Work out the finished part from the listing and answer in its coordinate system (mm). A direction names the side the tool comes from. Round coordinates to 2 decimals unless told otherwise and drop trailing zeros. Write each loop counter-clockwise with the first axis right and the second up, starting at its lowest first coordinate (ties: lowest second). Pieces come first, ordered by that corner, then holes.
1. A tool of negligible diameter and unlimited length cuts with its end or side. For faces 4 (the face through (-8.22, -54.25, 17.05)), 5 (the face through (5, -12, 10)), 6 (the face through (3, -33, 5.825)), 7 (the face through (10.07, -23.601, 13.605)), from which of +Z, -Z, +X, -X, +Y, -Y can it reach the whole face along a straight path? Write none if from no direction.
2. Find section B-B (x = -1.75). Write down the section's boundary in (y, z) (3 decimals), and give its area (3 significant figures).
3. Find section C-C (z = 10). Count the separate pieces of the cut face and the enclosed holes in it, and give its area (3 significant figures).
4. Flat-ended cylindrical pins translate along their axes: pin 1 Ø4 at (y, z) = (-57, 3) entering from -X; pin 2 Ø5 at (x, y) = (11.5, -12.5) entering from -Z; pin 3 Ø2.5 at (y, z) = (-57, 10.5) entering from -X; pin 4 Ø3.5 at (x, z) = (8.5, 10.5) entering from -Y. Find the tip coordinate at first contact, or state that the pin passes through.
5. Find section A-A (y = -24). Write down the section's boundary in (x, z) (3 decimals), and give its area (3 significant figures).
6. Determine the mould class of faces 1 (the face through (3, -33, 0)), 2 (the face through (-9, -21, 17)), 3 (the face through (10.07, -55.399, 13.605)) for opening direction Z: pulls with the +Z half, pulls with the -Z half, needs draft (parallel to the pull), parting line crosses it, or undercut.
7. Find section D-D (y = -50). Write down the section's boundary in (x, z) (3 decimals).
8. Straight lines are drawn through the part: probe 1 along Z at (x, y) = (8.2, -3); probe 2 along Z at (x, y) = (4.75, -46) (3 decimals); probe 3 along Y at (x, z) = (-7.5, 16.5). For each, find the intervals that lie inside material, in ascending order.
```python
from build123d import *

# Parameters (mm, degrees)
SKETCH_1_R          = 1.7
EXTRUDE_1_DEPTH     = 20
SKETCH_2_W          = 31.643510299
SKETCH_2_H          = 8.35
CUT_EXTRUDE_1_DEPTH = 75.850374033
SKETCH_4_R          = 1.7
CUT_EXTRUDE_3_DEPTH = 73.237455658
FILLET_1_R          = 0.5
FILLET_2_R          = 2
SKETCH_5_W          = 3.571488154
SKETCH_5_H          = 19.286036032
CUT_EXTRUDE_4_DEPTH = 75.850374033
FILLET_3_R          = 1.5
SKETCH_6_W          = 14.583576629
SKETCH_6_H          = 57.679533687
CUT_EXTRUDE_5_DEPTH = 75.850374033
FILLET_4_R          = 10
SKETCH_7_W          = 8.35
SKETCH_7_H          = 33
CUT_EXTRUDE_6_DEPTH = 71.370448485
FILLET_5_R          = 2


# Some blends are built 0.0001 mm under size
with BuildPart() as part:
    # 草图1 → 凸台-拉伸1 (new body)
    with BuildSketch(Plane.XY):
        with BuildLine():
            Line((0, 0), (10, 0))
            Line((10, 0), (10, -15))
            Line((10, -15), (29.096021943, -15))
            Line((29.096021943, -15), (29.096021943, -66))
            Line((29.096021943, -66), (-11.5, -66))
            Line((-11.5, -66), (-11.5, -54.4))
            ThreePointArc((-11.5, -54.4), (0.333421668, -43.75703287), (-9, -30.865568342))
            Line((-9, -30.865568342), (-9, -9.911704997))
            Line((-9, -9.911704997), (-7.763036189, -9.911704997))
            Line((-7.763036189, -9.911704997), (0, -4.543101007))
            Line((0, -4.543101007), (0, 0))
        make_face()
        with Locations((19.5, -30.6)):
            Circle(SKETCH_1_R, mode=Mode.SUBTRACT)
        with Locations((19.5, -56)):
            Circle(SKETCH_1_R, mode=Mode.SUBTRACT)
    extrude(amount=EXTRUDE_1_DEPTH)

    # 草图2 → 切除-拉伸1 (cut, through all)
    with BuildSketch(Plane(origin=(0, 0, 0), x_dir=(1, 0, 0), z_dir=(0, 1, 0))):
        with Locations((-10.82175515, -10)):
            Rectangle(SKETCH_2_W, SKETCH_2_H)
    extrude(amount=-CUT_EXTRUDE_1_DEPTH, mode=Mode.SUBTRACT)

    # 草图4 → 切除-拉伸3 (cut, through all)
    with BuildSketch(Plane(origin=(10, 0, 0), x_dir=(0, 0, -1), z_dir=(1, 0, 0))):
        with Locations(Location((-10, -3, 0), (0, 0, 90))):
            Circle(SKETCH_4_R)
        with Locations(Location((-10, -10, 0), (0, 0, 90))):
            Circle(SKETCH_4_R)
    extrude(amount=-CUT_EXTRUDE_3_DEPTH, mode=Mode.SUBTRACT)

    # 圆角1
    fillet_1_edges = [part.edges().sort_by_distance(p)[0] for p in [
        (-11.5, -66, 17.0875),
        (-9, -30.865568342, 17.0875),
        (-11.5, -66, 2.9125),
        (-9, -30.865568342, 2.9125),
    ]]
    fillet(fillet_1_edges, radius=FILLET_1_R)

    # 圆角2
    # the kernel refuses this fillet: 2 mm, written as the material it adds along each edge
    with BuildSketch(Plane(origin=(0, -4.543101007, 14.175), x_dir=(0, 1, 0), z_dir=(0, 0, 1)), Plane(origin=(0, -4.543101007, 0), x_dir=(0, 1, 0), z_dir=(0, 0, 1))) as fillet_2_piece_1:
        with BuildLine():
            CenterArc((FILLET_2_R * 0.524275273185, FILLET_2_R), FILLET_2_R, 214.666177241, 55.333822759)
            Line((-FILLET_2_R * 0.298204680815, FILLET_2_R * 0.431205902572), (0, 0))
            Line((0, 0), (FILLET_2_R * 0.524275273185, 0))
        make_face()
    extrude(amount=5.825)
    with BuildSketch(Plane(origin=(10, -15, 0), x_dir=(1, 0, 0), z_dir=(0, 0, 1))) as fillet_2_piece_2:
        with BuildLine():
            CenterArc((FILLET_2_R, FILLET_2_R), FILLET_2_R, 180, 90)
            Line((0, FILLET_2_R), (0, 0))
            Line((0, 0), (FILLET_2_R, 0))
        make_face()
    extrude(amount=20)
    # the kernel refuses this fillet: 2 mm, written as the material it takes off along each edge
    with BuildSketch(Plane(origin=(-9, -9.911704997, -4.621806853), x_dir=(0, -1, 0), z_dir=(0, 0, 1)), Plane(origin=(-9, -9.911704997, 9.553193147), x_dir=(0, -1, 0), z_dir=(0, 0, 1))) as fillet_2_2_piece_1:
        with BuildLine():
            CenterArc((1.848722741, 2), FILLET_2_R, 202.427748684, 67.572251316)
            Line((0, 1.236963811), (0, 0))
            Line((0, 0), (1.848722741, 0))
        make_face()
    extrude(amount=15.068613706, mode=Mode.SUBTRACT)
    with BuildSketch(Plane(origin=(0, 0, -5), x_dir=(1, 0, 0), z_dir=(0, 0, 1)), Plane(origin=(0, 0, 9.175), x_dir=(1, 0, 0), z_dir=(0, 0, 1))) as fillet_2_2_piece_2:
        with BuildLine():
            CenterArc((FILLET_2_R, -FILLET_2_R), FILLET_2_R, 90, 90)
            Line((0, -FILLET_2_R), (0, 0))
            Line((0, 0), (FILLET_2_R, 0))
        make_face()
    extrude(amount=15.825, mode=Mode.SUBTRACT)
    with BuildSketch(Plane(origin=(29.096021943, -15, -5), x_dir=(0, -1, 0), z_dir=(0, 0, 1)), Plane(origin=(29.096021943, -66, -5), x_dir=(-1, 0, 0), z_dir=(0, 0, 1))) as fillet_2_2_piece_3:
        with BuildLine():
            CenterArc((FILLET_2_R, -FILLET_2_R), FILLET_2_R, 90, 90)
            Line((0, -FILLET_2_R), (0, 0))
            Line((0, 0), (FILLET_2_R, 0))
        make_face()
    extrude(amount=30, mode=Mode.SUBTRACT)

    # 草图5 → 切除-拉伸4 (cut, through all)
    with BuildSketch(Plane.XY.offset(20)):
        with Locations((-10.285744077, -57.827803492)):
            Rectangle(SKETCH_5_W, SKETCH_5_H)
    extrude(amount=-CUT_EXTRUDE_4_DEPTH, mode=Mode.SUBTRACT)

    # 圆角3
    fillet_3_edges = [part.edges().sort_by_distance(p)[0] for p in [
        (-8.5, -54.015641537, 2.9125),
        (-8.5, -66, 2.9125),
        (-8.5, -54.015641537, 17.0875),
        (-8.5, -66, 17.0875),
    ]]
    fillet(fillet_3_edges, radius=FILLET_3_R)

    # 草图6 → 切除-拉伸5 (cut, through all)
    with BuildSketch(Plane(origin=(0, 0, 0), x_dir=(-1, 0, 0), z_dir=(0, 0, -1))):
        with Locations((-22.291788315, -40.000125123)):
            Rectangle(SKETCH_6_W, SKETCH_6_H)
    extrude(amount=-CUT_EXTRUDE_5_DEPTH, mode=Mode.SUBTRACT)

    # 圆角4
    fillet_4_edges = [part.edges().sort_by_distance(p)[0] for p in [
        (15, -66, 10),
        (15, -15, 10),
    ]]
    fillet(fillet_4_edges, radius=FILLET_4_R - 0.0001)  # a hair under: the kernel refuses the full size

    # 草图7 → 切除-拉伸6 (cut, through all)
    with BuildSketch(Plane.ZY.offset(-5)):
        with Locations((10, -39.5)):
            Rectangle(SKETCH_7_W, SKETCH_7_H)
    extrude(amount=-CUT_EXTRUDE_6_DEPTH, mode=Mode.SUBTRACT)

    # 圆角5
    fillet_5_edges = [part.edges().sort_by_distance(p)[0] for p in [
        (10, -56, 5.825),
        (10, -23, 5.825),
        (10, -23, 14.175),
        (10, -56, 14.175),
    ]]
    fillet(fillet_5_edges, radius=FILLET_5_R)


solid = part.part
```
Worked answers:
1. face 4: +Z, -Z, -X
1. face 5: -X, +Y, -Y
1. face 6: -X
1. face 7: +X, -X
2. outline: (-66, 0) - (-49.323, 0) - (-49.323, 5.825) - (-66, 5.825) - close; (-66, 14.175) - (-49.323, 14.175) - (-49.323, 20) - (-66, 20) - close; (-35.677, 0) - (-5.753, 0) - (-5.753, 5.825) - (-35.677, 5.825) - close; (-35.677, 14.175) - (-5.753, 14.175) - (-5.753, 20) - (-35.677, 20) - close
2. area: 543 mm2
3. separate pieces: 4
3. enclosed holes: 0
3. area: 192 mm2
4. pin 1: stops at x = -8.5
4. pin 2: stops at z = 0
4. pin 3: stops at x = 5
4. pin 4: stops at y = -65.85
5. outline: (-9, 0) - (15, 0) - (15, 6.093) - (5, 6.093) - (5, 5.825) - (-9, 5.825) - close; (-9, 14.175) - (5, 14.175) - (5, 13.907) - (15, 13.907) - (15, 20) - (-9, 20) - close
5. area: 285 mm2
6. face 1: pulls with the -Z half
6. face 2: needs draft
6. face 3: undercut
7. outline: (-2.261, 0) - (15, 0) - (15, 5.825) - (-2.261, 5.825) - close; (-2.261, 14.175) - (15, 14.175) - (15, 20) - (-2.261, 20) - close
8. probe 1: z = 0 to 8.3, 11.7 to 20
8. probe 2: z = 0 to 5.825, 14.175 to 20
8. probe 3: y = -65.91 to -53.71, -31.29 to -9.73
